```python
from build123d import *

# Parameters (mm, degrees)
F0_R     = 22.9235
F1_DEPTH = 3.6576
F2_R     = 2.54
F3_DEPTH = 3.6586
F2_R_2   = 1.524
F4_DEPTH = 25.4
F5_R     = 2.921
F5_R_2   = 1.524
F6_DEPTH = 1.905


# Not quite as in the source:
# - a feature names something its author has since deleted; it is built from what else it names


with BuildPart() as f1:
    # F0 (on Top) → F1 (new body)
    with BuildSketch(Plane.XY):
        Circle(F0_R)
    extrude(amount=F1_DEPTH)

    # F2 (on face) → F3 (cut, through all)
    with BuildSketch(Plane.XY.offset(3.6576)):
        with Locations((0, -19.1135)):
            Circle(F2_R)
        with Locations((0, -12.7635)):
            Circle(F2_R)
    extrude(amount=-F3_DEPTH, mode=Mode.SUBTRACT)

    # F2 (on face) → F4 (cut)
    with BuildSketch(Plane.XY.offset(3.6576)):
        Circle(F2_R_2)
    extrude(amount=-F4_DEPTH, mode=Mode.SUBTRACT)

    # F5 (on face) → F6 (cut)
    with BuildSketch(Plane.XY.offset(3.6576)):
        Circle(F5_R)
        Circle(F5_R_2, mode=Mode.SUBTRACT)
    extrude(amount=-F6_DEPTH, mode=Mode.SUBTRACT)


solid = f1.part
```
Geometry: final body of the model. Coordinates: model frame, mm. A direction names the side the tool comes from. Coordinates: 2 decimals unless noted, no trailing zeros. Order: outer loops, then holes, each group sorted by start corner. A loop starts at its lowest first (then second) coordinate and runs counter-clockwise, first axis right, second up. Notation, with made-up numbers: (68, 38) -> (114, 38) arc R16 ccw to (114, 68) -> close; hole circle Ø11 at (16, 70). An arc over 180 degrees is marked (long way). Write item = value, one per line.
(1) Cut plane A-A on y = 0. Return loops of the section in (x, z), plus the area to 3 significant figures.
Solved:
outline = (-22.92, 0) -> (-1.52, 0) -> (-1.52, 1.75) -> (-2.92, 1.75) -> (-2.92, 3.66) -> (-22.92, 3.66) -> close; (1.52, 0) -> (22.92, 0) -> (22.92, 3.66) -> (2.92, 3.66) -> (2.92, 1.75) -> (1.52, 1.75) -> close
area = 151 mm²
(2) Access query for faces 1 (the cylindrical face through (-0.2, 1.51, 0.89)), 2 (the flat face through (1.3, -1.3, 1.753)). Directions: +Z, -Z, +X, -X, +Y, -Y. A direction counts if a zero-diameter tool reaches every point of the face in a straight line with its end or side. Return the directions, or none.
Solved:
face_1 = +Z, -Z
face_2 = +Z
(3) Cut plane B-B on x = 0. Return loops of the section in (y, z).
Solved:
outline = (-22.92, 0) -> (-21.65, 0) -> (-21.65, 3.66) -> (-22.92, 3.66) -> close; (-16.57, 0) -> (-15.3, 0) -> (-15.3, 3.66) -> (-16.57, 3.66) -> close; (-10.22, 0) -> (-1.52, 0) -> (-1.52, 1.75) -> (-2.92, 1.75) -> (-2.92, 3.66) -> (-10.22, 3.66) -> close; (1.52, 0) -> (22.92, 0) -> (22.92, 3.66) -> (2.92, 3.66) -> (2.92, 1.75) -> (1.52, 1.75) -> close
(4) Cut plane D-D on x = -18. Return loops of the section in (y, z), plus the area to 3 significant figures.
Solved:
outline = (-14.19, 0) -> (14.19, 0) -> (14.19, 3.66) -> (-14.19, 3.66) -> close
area = 104 mm²
(5) Cut plane C-C on y = -14. Return loops of the section in (x, z).
Solved:
outline = (-18.15, 0) -> (-2.22, 0) -> (-2.22, 3.66) -> (-18.15, 3.66) -> close; (2.22, 0) -> (18.15, 0) -> (18.15, 3.66) -> (2.22, 3.66) -> close
(6) Pin query (flat end, axial travel): pin 1 Ø1 at (x, z) = (-13.5, 2) entering from -Y; pin 2 Ø1 at (y, z) = (1, 2.5) entering from +X; pin 3 Ø3 at (x, y) = (1, 0.5) entering from +Z. Return the tip coordinate at first contact, or that it passes through.
Solved:
pin_1 = -18.88
pin_2 = 22.92
pin_3 = 1.75
(7) Line query: line 1 (Y direction, x = 0, z = 0.5); line 2 (Y direction, x = 0, z = 2.3); line 3 (X direction, y = -12, z = 2.65). Output: solid intervals per line, ascending.
Solved:
line_1 = -22.92 to -21.65, -16.57 to -15.3, -10.22 to -1.52, 1.52 to 22.92
line_2 = -22.92 to -21.65, -16.57 to -15.3, -10.22 to -2.92, 2.92 to 22.92
line_3 = -19.53 to -2.42, 2.42 to 19.53
(8) Pull-direction query (X, two-part tool) for faces 3 (the cylindrical face through (-2.98, 22.73, 1.8)), 4 (the flat face through (5, 0, 3.658)), 5 (the cylindrical face through (-0.551, -15.243, 1.854)); classes: pulls with the +X half, pulls with the -X half, needs draft (parallel to the pull), parting line crosses it, or undercut.
Solved:
face_3 = parting line crosses it
face_4 = needs draft
face_5 = undercut
